Study the drawing (mm; zero at the part's minimum x, y, z) and answer. A direction names the side the tool comes from. Round coordinates to 2 decimals unless told otherwise and drop trailing zeros. Write each loop counter-clockwise with the first axis right and the second up, starting at its lowest first coordinate (ties: lowest second). Pieces come first, ordered by that corner, then holes.
(1) A cutting plane is placed at B-B, the plane z = 4. Give the vertices of the cut face in (x, y).
(2) Each of these flat-tipped pins is pushed along its axis until it touches: pin 1 Ø2 at (y, z) = (2.5, 5) entering from +X; pin 2 Ø0.9 at (x, y) = (9, 4) entering from -Z; pin 3 Ø2.5 at (x, z) = (4, 4) entering from -Y; pin 4 Ø3 at (x, z) = (7, 7) entering from +Y. Where does it stop, or does it pass through?
(3) A cutting plane is placed at D-D, the plane x = 13.75. Give the vertices of the cut face in (y, z).
(4) A cutting plane is placed at A-A, the plane x = 11. Give the vertices of the cut face in (y, z).
(5) Find the intervals of material crossed by probe 1 along Y at (x, z) = (11.75, 6.75); probe 2 along X at (y, z) = (1.3, 4.25); probe 3 along Z at (x, y) = (7.75, 3.2), in increasing order.
(6) The mould has two halves that part along X. Classify the marked faces 1, 2 and 3: +X half, -X half, draft (parallel to the pull), parting line (faces both ways), or undercut.
(7) For the marked faces 4 and 5, determine the directions among +Z, -Z, +X, -X, +Y, -Y from which every point of the face is accessible in a straight line to the end or side of a thin tool.
(8) A cutting plane is placed at C-C, the plane y = 3.6. Give the vertices of the cut face in (x, z).
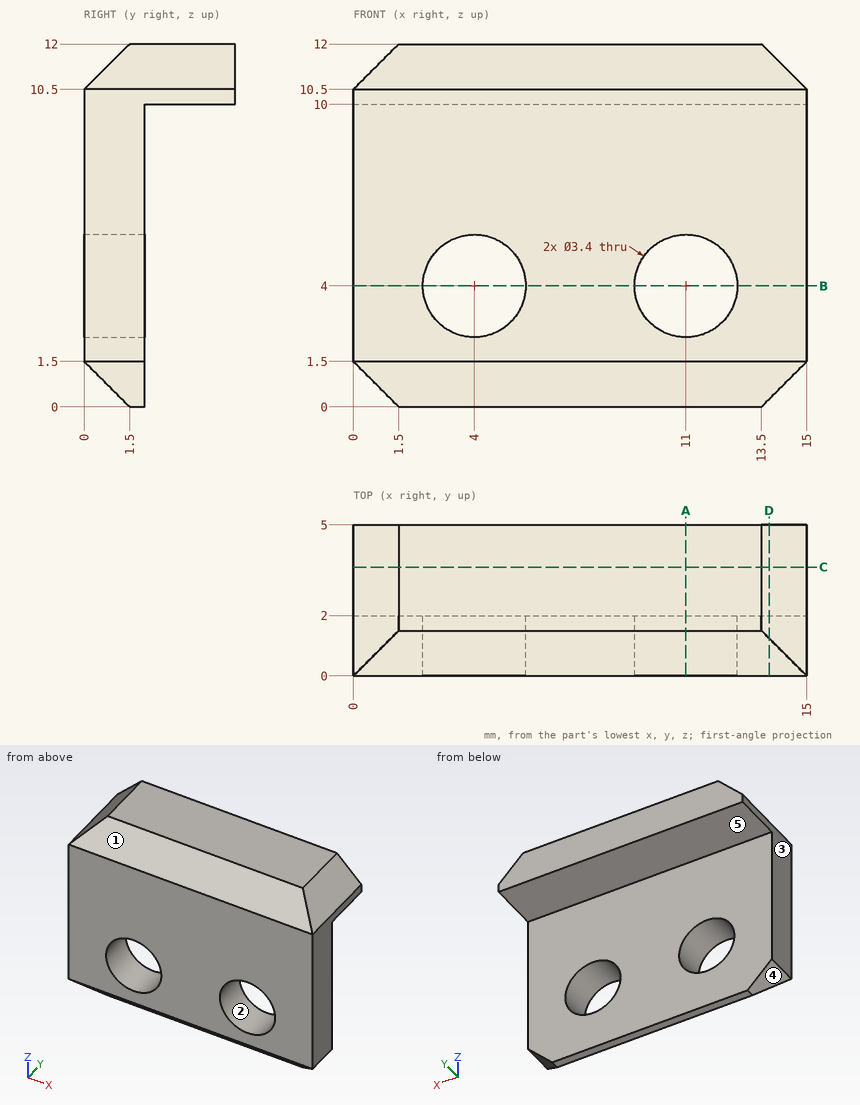
Solutions:
1. outline: (0, 0) - (2.3, 0) - (2.3, 2) - (0, 2) - close; (5.7, 0) - (9.3, 0) - (9.3, 2) - (5.7, 2) - close; (12.7, 0) - (15, 0) - (15, 2) - (12.7, 2) - close
2. pin 1: stops at x = 15
2. pin 2: stops at z = 10
2. pin 3: passes through
2. pin 4: stops at y = 2
3. outline: (0, 1.5) - (1.25, 0.25) - (2, 0.25) - (2, 10) - (5, 10) - (5, 11.75) - (1.25, 11.75) - (0, 10.5) - close
4. outline: (0, 1.5) - (1.5, 0) - (2, 0) - (2, 2.3) - (0, 2.3) - close; (0, 5.7) - (2, 5.7) - (2, 10) - (5, 10) - (5, 12) - (1.5, 12) - (0, 10.5) - close
5. probe 1: y = 0 to 2
5. probe 2: x = 0 to 2.32, 5.68 to 9.32, 12.68 to 15
5. probe 3: z = 10 to 12
6. face 1: draft
6. face 2: undercut
6. face 3: -X half
7. face 4: -Z, -X, +Y, -Y
7. face 5: -Z, +X, -X, +Y
8. outline: (0, 10) - (15, 10) - (15, 10.5) - (13.5, 12) - (1.5, 12) - (0, 10.5) - close
